from build123d import *

# Parameters (mm, degrees)
BOSS_EXTRUDE1_DEPTH = 1.5
SKETCH3_W           = 1
SKETCH3_H           = 3.5
CUT_EXTRUDE2_DEPTH  = 1.5


with BuildPart() as part:
    # Sketch1 → Boss-Extrude1 (new body)
    with BuildSketch(Plane.XY):
        with BuildLine():
            Line((-4.539904997, -8.910065242), (-7.944833745, -15.592614173))
            ThreePointArc((-7.944833745, -15.592614173), (0, 17.5), (7.944833745, -15.592614173))
            Line((7.944833745, -15.592614173), (4.539904997, -8.910065242))
            ThreePointArc((4.539904997, -8.910065242), (0, 10), (-4.539904997, -8.910065242))
        make_face()
    extrude(amount=BOSS_EXTRUDE1_DEPTH)

    # Sketch3 → Cut-Extrude2 (cut)
    with BuildSketch(Plane.XY.offset(1.5)):
        Polygon((-13.448841764, -3.075278615), (-11.948841764, -3.075278615), (-11.948841764, -6.575278615), (-13.448841764, -6.575278615), (-13.448841764, -5.700278615), (-12.594138864, -5.700278615), (-12.594138864, -5.200278615), (-13.448841764, -5.200278615), (-13.448841764, -4.450278615), (-12.594138864, -4.450278615), (-12.594138864, -3.950278615), (-13.448841764, -3.950278615), align=None)
        Polygon((-6.189760479, 13.023085903), (-6.189760479, 9.523085903), (-7.689760479, 9.523085903), (-7.689760479, 10.023085903), (-6.689760479, 10.023085903), (-6.689760479, 10.523085903), (-6.689760479, 12.259445402), (-7.189760479, 12.259445402), (-7.189760479, 11.523085903), (-6.989760479, 11.523085903), (-6.989760479, 11.023085903), (-7.189760479, 11.023085903), (-7.689760479, 11.023085903), (-7.689760479, 13.023085903), align=None)
        with Locations((8.681961549, 9.557519934)):
            Rectangle(SKETCH3_W, SKETCH3_H)
        Polygon((10.181961549, 11.307519934), (10.181961549, 9.307519934), (10.681961549, 9.307519934), (10.681961549, 8.807519934), (10.181961549, 8.807519934), (10.181961549, 7.807519934), (11.681961549, 7.807519934), (11.681961549, 9.807519934), (11.181961549, 9.807519934), (11.181961549, 10.307519934), (11.681961549, 10.307519934), (11.681961549, 11.307519934), align=None)
        with Locations((12.435856983, -7.53707486)):
            Rectangle(SKETCH3_W, SKETCH3_H)
        Polygon((9.435856983, -5.78707486), (10.935856983, -5.78707486), (10.935856983, -7.78707486), (10.435856983, -7.78707486), (10.435856983, -8.28707486), (10.935856983, -8.28707486), (10.935856983, -9.28707486), (9.435856983, -9.28707486), (9.435856983, -7.285099387), (9.935856983, -7.285099387), (9.935856983, -6.78707486), (9.435856983, -6.78707486), align=None)
        Polygon((-9.472185157, -6.970667712), (-10.030119205, -6.14078242), (-7.540463329, -4.466980276), (-6.982529281, -5.296865568), align=None)
        Polygon((-5.606922021, -6.736091259), (-6.337757985, -6.053538116), (-8.385417415, -8.246046009), (-7.654581451, -8.928599152), align=None)
        Polygon((-11.001594478, 4.156611473), (-12.900873876, 4.783299409), (-13.214217844, 3.83365971), (-11.314938446, 3.206971774), (-8.466019349, 2.26693987), (-8.152675381, 3.216579569), align=None)
        Polygon((1.831331602, 11.617173691), (2.058491975, 13.604231356), (1.064963142, 13.717811542), (0.83780277, 11.730753877), (0.497062212, 8.750167379), (1.490591044, 8.636587193), align=None)
        Polygon((-11.572476541, -2.0953011), (-11.70864319, -1.104615154), (-8.736585352, -0.696115207), (-8.600418703, -1.686801153), align=None)
        Polygon((-11.746785331, 0.570556211), (-11.655850469, 1.566413053), (-8.668279941, 1.293608466), (-8.759214803, 0.297751624), align=None)
        Polygon((-10.299219978, 5.677901711), (-9.779636028, 6.532321115), (-7.216377815, 4.973569265), (-7.735961765, 4.119149861), align=None)
        Polygon((-8.752042864, 7.855841502), (-8.053030417, 8.570951003), (-5.907701913, 6.473913662), (-6.60671436, 5.758804161), align=None)
        Polygon((11.746785331, 0.570556211), (13.738499016, 0.752425935), (13.647564154, 1.748282778), (11.655850469, 1.566413053), (8.668279941, 1.293608466), (8.759214803, 0.297751624), align=None)
        Polygon((-4.405965904, 10.904126029), (-3.463704982, 11.239005641), (-2.459066145, 8.412222875), (-3.401327068, 8.077343262), align=None)
        Polygon((-1.831331602, 11.617173691), (-0.83780277, 11.730753877), (-0.497062212, 8.750167379), (-1.490591044, 8.636587193), align=None)
        Polygon((3.463704982, 11.239005641), (4.405965904, 10.904126029), (3.401327068, 8.077343262), (2.459066145, 8.412222875), align=None)
        Polygon((5.910873662, 10.167304094), (6.753244282, 9.628405458), (5.136548374, 7.101293601), (4.294177755, 7.640192237), align=None)
        Polygon((9.779636028, 6.532321115), (10.299219978, 5.677901711), (7.735961765, 4.119149861), (7.216377815, 4.973569265), align=None)
        Polygon((11.001594478, 4.156611473), (11.314938446, 3.206971774), (8.466019349, 2.26693987), (8.152675381, 3.216579569), align=None)
        Polygon((11.70864319, -1.104615154), (11.572476541, -2.0953011), (8.600418703, -1.686801153), (8.736585352, -0.696115207), align=None)
        Polygon((11.157248442, -3.718643193), (10.801006731, -4.65303703), (7.997825219, -3.584311895), (8.354066931, -2.649918058), align=None)
        Polygon((8.385417415, -8.246046009), (7.654581451, -8.928599152), (5.606922021, -6.736091259), (6.337757985, -6.053538116), align=None)
    extrude(amount=-CUT_EXTRUDE2_DEPTH, mode=Mode.SUBTRACT)


solid = part.part
Can you work these out from the model? Positions are in its coordinate system, mm. A direction names the side the tool comes from. Give positions to 0.01 mm unless a question says otherwise; leave off trailing zeros. Order: outer loops, then holes, each group sorted by start corner. A loop starts at its lowest first (then second) coordinate and runs counter-clockwise, first axis right, second up. Notation, with made-up numbers: M -32.5,-0.75 L 13.5,-0.75 A24 ccw 13.5,33.25 Z; hole C 6,84 d8. An arc over 180 degrees is marked long. Use a Markdown table: item, result. Add a question column.
Item 1: If I drill on L1, parallel to X at y = -8, z = 1.2; L2, parallel to Y at x = 9, z = 0.25; L3, parallel to X at y = -7.5, z = 0.1, over which ranges is the centre line in solid material (lowest first)? Write a range as [from, to].
Item 2: Suppose I cut it at B-B (z = 1.2). Count the separate pieces of the cut face and the enclosed holes in it, then the cut area to 3 significant figures.
Item 3: We'd pull the mould along Y, two halves only. Please class faces 1 (the cylindrical face through (-0.654, 17.488, 0.74)), 2 (the flat face through (-7, 13.023, 1)), 3 (the flat face through (-3.173, 10.42, 0.76)): +Y half, -Y half, draft (parallel to the pull), parting line (faces both ways), or undercut.
Item 4: Will these pins go through, and if not, where does the flat tip stop? pin 1 (0.8 mm diameter, centred on y = -7.5, z = 1, fed in from -X) (3 decimals); pin 2 (0.6 mm diameter, centred on x = 10.5, z = 1, fed in from -Y); pin 3 (0.5 mm diameter, centred on x = 12.5, z = 0.5, fed in from +Y); pin 4 (4 mm diameter, centred on x = 6.5, y = -4.5, fed in from +Z).
Item 5: Suppose I cut it at C-C (x = 0). List the corners of the cut face in (y, z) for me.
Item 6: For faces 4 (the flat face through (6.266, -12.298, 0.74)), 5 (the cylindrical face through (8, -6, 1)), which set-ups out of +Z, -Z, +X, -X, +Y, -Y let a thin tool reach every point of the face, with its end or its side?
Item 7: Suppose I cut it at A-A (y = 0). List the corners of the cut face in (x, z) for me.
Answer sheet:
| question | item | result |
|---|---|---|
| 1 | L1 | x = [-15.56, -8.16], [-6.79, -6], [6, 6.79], [8.16, 9.44], [10.44, 11.94], [12.94, 15.56] |
| 1 | L2 | y = [-15.01, -4.36], [4.36, 4.89], [6.06, 7.81], [11.31, 15.01] |
| 1 | L3 | x = [-15.81, -7.69], [7.69, 9.44], [10.94, 11.94], [12.94, 15.81] |
| 2 | separate pieces | 1 |
| 2 | enclosed holes | 6 |
| 2 | area | 489 mm² |
| 3 | face 1 | parting line |
| 3 | face 2 | undercut |
| 3 | face 3 | -Y half |
| 4 | pin 1 | stops at x = -15.995 |
| 4 | pin 2 | stops at y = -14.22 |
| 4 | pin 3 | stops at y = 12.5 |
| 4 | pin 4 | passes through |
| 5 | outline | M 10,0 L 17.5,0 L 17.5,1.5 L 10,1.5 Z |
| 6 | face 4 | +Z, -Z, -Y |
| 6 | face 5 | +Z, -Z |
| 7 | outline | M -17.5,0 L -10,0 L -10,1.5 L -17.5,1.5 Z; M 10,0 L 17.5,0 L 17.5,1.5 L 10,1.5 Z |
